```python
from build123d import *

# Parameters (mm, degrees)
F0_W     = 25.4
F0_H     = 19.05
F0_H_2   = 4.7498
F0_H_3   = 4.7752
F1_DEPTH = 63.5


with BuildPart() as f1:
    # F0 (on Front) → F1 (new body, symmetric)
    with BuildSketch(Plane.XZ):
        Polygon((-41.275, -9.525), (41.275, -9.525), (41.275, 0), (41.275, 9.525), (22.225, 9.525), (-41.275, 9.525), align=None)
        with BuildLine():
            add(Edge.make_bspline(
                [(-41.275, 9.525), (-40.1127492215, 45.3608282082), (10.2455717383, 58.7983861186), (51.8289972112, 61.5174790689)],
                knots=[0, 0, 0, 0, 106.414059963, 106.414059963, 106.414059963, 106.414059963], degree=3))
            Line((-41.275, 9.525), (22.225, 9.525))
            Line((22.225, 9.525), (22.225, 27.0002))
            ThreePointArc((22.225, 27.0002), (30.63970344, 49.7369500162), (51.8289972112, 61.5174790689))
        make_face()
        with BuildLine():
            Line((22.225, 9.525), (41.275, 9.525))
            Line((41.275, 9.525), (41.275, 27.0002))
            ThreePointArc((41.275, 27.0002), (45.9246798487, 38.2255201513), (57.15, 42.8752))
            Line((57.15, 42.8752), (76.2, 42.8752))
            Line((76.2, 42.8752), (76.2, 61.9252))
            Line((76.2, 61.9252), (60.1124922335, 61.9252))
            add(Edge.make_bspline(
                [(51.8289972112, 61.5174790689), (54.6360932505, 61.7010318899), (57.4032025523, 61.8357412294), (60.1124922335, 61.9252)],
                knots=[106.414059963, 106.414059963, 106.414059963, 106.414059963, 113.5975587454, 113.5975587454, 113.5975587454, 113.5975587454], degree=3))
            ThreePointArc((51.8289972112, 61.5174790689), (30.63970344, 49.7369500162), (22.225, 27.0002))
            Line((22.225, 27.0002), (22.225, 9.525))
        make_face()
        with BuildLine():
            ThreePointArc((57.15, 61.9252), (54.4816996498, 61.8231205875), (51.8289972112, 61.5174790689))
            add(Edge.make_bspline(
                [(51.8289972112, 61.5174790689), (54.6360932505, 61.7010318899), (57.4032025523, 61.8357412294), (60.1124922335, 61.9252)],
                knots=[106.414059963, 106.414059963, 106.414059963, 106.414059963, 113.5975587454, 113.5975587454, 113.5975587454, 113.5975587454], degree=3))
            Line((60.1124922335, 61.9252), (57.15, 61.9252))
        make_face()
        with BuildLine():
            add(Edge.make_bspline(
                [(60.1124922335, 61.9252), (65.7827499857, 62.1124277781), (71.1997457835, 62.1014486601), (76.2, 61.9252)],
                knots=[113.5975587454, 113.5975587454, 113.5975587454, 113.5975587454, 128.6318645789, 128.6318645789, 128.6318645789, 128.6318645789], degree=3))
            Line((60.1124922335, 61.9252), (76.2, 61.9252))
        make_face()
        with Locations((88.9, 52.4002)):
            Rectangle(F0_W, F0_H)
        with Locations((88.9, 64.3001)):
            Rectangle(F0_W, F0_H_2)
        with Locations((88.9, 40.4876)):
            Rectangle(F0_W, F0_H_3)
        Polygon((101.6, 66.675), (101.6, 61.9252), (101.6, 42.8752), (101.6, 38.1), (127, 38.1), (127, 66.675), align=None)
    extrude(amount=F1_DEPTH, both=True)


solid = f1.part
```
Source: CAD feature listing. Evaluate the final solid. Frame: model axes, mm. A direction names the side the tool comes from. Round coordinates to 2 decimals unless told otherwise and drop trailing zeros. Loops run counter-clockwise (first coordinate to the right, second up) from the corner with the lowest first, then second, coordinate; pieces in that order, holes last. Notation, with made-up numbers: M 10.25,10 L 32.25,10 A19 ccw 32.25,28 Z; hole C 60.25,40.25 d3. An arc over 180 degrees is marked long. Use a Markdown table: item, result. Add a question column.
1. Line query: line 1 (X direction, y = 49, z = 62.5); line 2 (Z direction, x = 65, y = 50); line 3 (Z direction, x = 116, y = -50) (3 decimals). Output: solid intervals per line, ascending.
2. Reachability of faces 1 (the flat face through (41.275, -1, 8)), 2 (the flat face through (102, -1, 66.675)), 3 (the flat face through (76.2, -1, 40)) from +Z, -Z, +X, -X, +Y, -Y: full face, straight path, thin tool, end or side. Return the list, or none.
3. Contact query for flat-ended pins moving along their axis: P1, Ø2.5, axis at y = 15.5, z = 40, coming from the -X side; P2, Ø18.5, axis at y = -26, z = 2.5, coming from the +X side (3 decimals); P3, Ø1.5, axis at x = 67, y = 6, coming from the +Z side. Output: stop coordinate, or through.
4. Section query A-A on x = 112.5. Return the cut outline in (y, z) (3 decimals).
5. Section query B-B on z = 7. Return the cut outline in (x, y) (3 decimals).
Reported:
| question | item | result |
|---|---|---|
| 1 | line 1 | x = 76.2 to 127 |
| 1 | line 2 | z = 42.88 to 62.04 |
| 1 | line 3 | z = 38.1 to 66.675 |
| 2 | face 1 | -Z, +X, +Y, -Y |
| 2 | face 2 | +Z, +X, -X, +Y, -Y |
| 2 | face 3 | -Z, +Y, -Y |
| 3 | P1 | stops at x = -25.33 |
| 3 | P2 | stops at x = 41.275 |
| 3 | P3 | stops at z = 62.06 |
| 4 | outline | M -63.5,38.1 L 63.5,38.1 L 63.5,66.675 L -63.5,66.675 Z |
| 5 | outline | M -41.275,-63.5 L 41.275,-63.5 L 41.275,63.5 L -41.275,63.5 Z |
